Source: three-view drawing plus pictorial views. Frame: mm from the lowest corner of the part. A direction names the side the tool comes from. Round coordinates to 2 decimals unless told otherwise and drop trailing zeros. Order: outer loops, then holes, each group sorted by start corner. A loop starts at its lowest first (then second) coordinate and runs counter-clockwise, first axis right, second up. Notation, with made-up numbers: (60, 42) - (105, 42) arc R30 ccw to (105, 66) - close; hole circle Ø6 at (11.25, -3.75). An arc over 180 degrees is marked (long way). Use one line per item in the form item = value. Start each with the question number.
Q1. Cut plane B-B, the plane z = 15. Return the cut outline in (x, y), and give its area (3 significant figures).
Q2. Cut plane C-C, the plane y = 3.5. Return the cut outline in (x, z).
Q3. Draft query along Z for the marked faces 4, 5, 6 and 7. Return one class per face: released by +Z, released by -Z, zero draft, split by the parting line, or undercut.
Q4. Cut plane D-D, the plane z = 8.5. Return the cut outline in (x, y), and give its area (3 significant figures).
Q5. Cut plane A-A, the plane x = 9. Return the cut outline in (y, z), and give its area (3 significant figures).
Q6. Pin query (flat end, axial travel): pin 1 Ø7 at (x, z) = (9, 15) entering from +Y; pin 2 Ø3.5 at (x, z) = (49, 15) entering from -Y. Return the tip coordinate at first contact, or that it passes through.
Q7. Ray query, line 1 (X direction, y = 2.5, z = 15); line 2 (Y direction, x = 7.5, z = 24); line 3 (X direction, y = 10.25, z = 14). Return the intervals inside material, ascending. Write a range as [from, to].
Q8. Set-up query: the marked faces 1, 2 and 3. Return all of +Z, -Z, +X, -X, +Y, -Y with unobstructed straight access to the full face (end or side cutting, diameter ignored); none if empty.
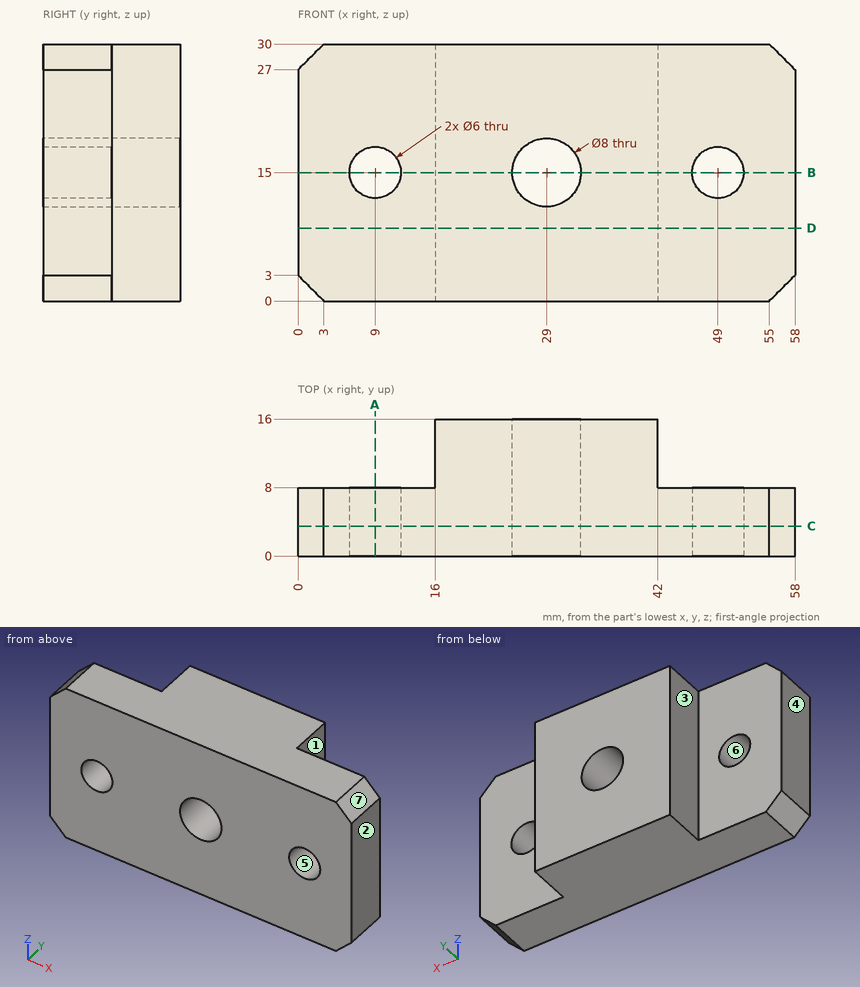
Completed:
q1.outline = (0, 0) - (6, 0) - (6, 8) - (0, 8) - close; (12, 0) - (25, 0) - (25, 16) - (16, 16) - (16, 8) - (12, 8) - close; (33, 0) - (46, 0) - (46, 8) - (42, 8) - (42, 16) - (33, 16) - close; (52, 0) - (58, 0) - (58, 8) - (52, 8) - close
q1.area = 448 mm2
q2.outline = (0, 3) - (3, 0) - (55, 0) - (58, 3) - (58, 27) - (55, 30) - (3, 30) - (0, 27) - close; hole circle Ø6 at (9, 15); hole circle Ø8 at (29, 15); hole circle Ø6 at (49, 15)
q3.face_4 = zero draft
q3.face_5 = undercut
q3.face_6 = undercut
q3.face_7 = released by +Z
q4.outline = (0, 0) - (58, 0) - (58, 8) - (42, 8) - (42, 16) - (16, 16) - (16, 8) - (0, 8) - close
q4.area = 672 mm2
q5.outline = (0, 0) - (8, 0) - (8, 12) - (0, 12) - close; (0, 18) - (8, 18) - (8, 30) - (0, 30) - close
q5.area = 192 mm2
q6.pin_1 = 8
q6.pin_2 = through
q7.line_1 = [0, 6], [12, 25], [33, 46], [52, 58]
q7.line_2 = [0, 8]
q7.line_3 = [16, 25.13], [32.87, 42]
q8.face_1 = +Z, -Z, +X, +Y
q8.face_2 = +Z, -Z, +X, +Y, -Y
q8.face_3 = +Z, -Z, -X, +Y
